Read the model definition and answer for the solid it produces. Units are mm, in the model's axes. A direction names the side the tool comes from. Give positions to 0.01 mm unless a question says otherwise; leave off trailing zeros. Loops run counter-clockwise (first coordinate to the right, second up) from the corner with the lowest first, then second, coordinate; pieces in that order, holes last. Notation, with made-up numbers: (36.5, 84.25) - (76.5, 84.25) arc R30 cw to (76.5, 122.25) - close; hole circle Ø6 at (82, 3.5). An arc over 180 degrees is marked (long way). Put each result on its own line as item: value. Start each with the question number.
1. A cutting plane is placed at C-C, the plane y = 5.5. Determine the outline of the cut face in (x, z), plus the area to 3 significant figures.
2. Consider L1, parallel to Z at x = 5, y = 1.5; L2, parallel to X at y = -0.5, z = 6; L3, parallel to X at y = -10.5, z = -11. Determine where each line is inside the solid, lowest interval first. Write a range as from..to.
3. A cutting plane is placed at D-D, the plane x = 13. Determine the outline of the cut face in (y, z), plus the area to 3 significant figures.
4. For faces 4 (the cylindrical face through (77.91, 0.21, -29.19)), 5 (the cylindrical face through (37.73, -0.07, 4.06)), 6 (the flat face through (23, -4, 0)), determine the directions among +Z, -Z, +X, -X, +Y, -Y from which every point of the face is accessible in a straight line to the end or side of a thin tool.
5. A cutting plane is placed at B-B, the plane y = 0. Determine the outline of the cut face in (x, z).
6. A cutting plane is placed at A-A, the plane x = 26.5. Determine the outline of the cut face in (y, z), plus the area to 3 significant figures.
7. Given pin 1 Ø2 at (y, z) = (-4.5, -28) entering from +X; pin 2 Ø3 at (x, y) = (59.5, -10) entering from -Z; pin 3 Ø5 at (y, z) = (-12, -5.5) entering from +X, each flat-ended and moving along its own axis, determine where each tip first touches the part or whether it passes through.
8. For a pull along X with two mould halves and no side action, classify faces 1 (the flat face through (60.66, -0.21, -17.47)), 2 (the flat face through (25, 3, 4)), 3 (the flat face through (43, -15, 2)) as released by +X, released by -X, zero draft, split by the parting line, or undercut.
```python
from build123d import *

# Parameters (mm, degrees)
F1_DEPTH    = 15
F3_DEPTH    = 43.4455230334
F5_D        = 4
F6_T1_DEPTH = 78.9897948557
F6_T3_DEPTH = 58
F7_SIZE     = 5


# Not quite as in the source:
# - a fillet or chamfer that OpenCascade refuses, or shapes differently, is made with other operations: its cross-section is extruded or revolved along the edge and cut away or added


with BuildPart() as f1:
    # F0 (on Front) → F1 (new body, symmetric)
    with BuildSketch(Plane.XZ):
        Polygon((-0.2695387348, 8), (0, 0), (46, 0), (75.7414862046, -35.4445230334), (81.8698417496, -30.3022221559), (49.7304612652, 8), align=None)
    extrude(amount=F1_DEPTH, both=True)

    # F2 (on face) → F3 (cut, through all)
    with BuildSketch(Plane.XY.offset(8)):
        with BuildLine():
            ThreePointArc((14.7304612652, 3), (11.7304612652, 0), (14.7304612652, -3))
            Line((14.7304612652, -3), (34.7304612652, -3))
            ThreePointArc((34.7304612652, -3), (37.7304612652, 0), (34.7304612652, 3))
            Line((34.7304612652, 3), (14.7304612652, 3))
        make_face()
    extrude(amount=-F3_DEPTH, mode=Mode.SUBTRACT)

    # F5 (through all)
    with Locations(Plane(origin=(33.1222636313, 0, 27.7928791968), x_dir=(0, 1, 0), z_dir=(0.7660444431, 0, 0.6427876097))):
        with Locations((0, -40.8377687803), (0, -60.8377687803)):
            Hole(F5_D / 2)

    # F6: fillet of radius 10 on 2 edges, made by hand

    # F6_s2 → F6_t1 (cut)
    with BuildSketch(Plane.XZ.offset(-39.4948974278)):
        with BuildLine():
            ThreePointArc((75.7414862046, -35.4445230334), (77.9104912295, -29.0903052725), (75.5718351227, -22.7965501322))
            Line((75.5718351227, -22.7965501322), (81.8698417496, -30.3022221559))
            Line((81.8698417496, -30.3022221559), (75.7414862046, -35.4445230334))
        make_face()
    extrude(amount=F6_T1_DEPTH, mode=Mode.SUBTRACT)

    # F6_s4 → F6_t3 (cut)
    with BuildSketch(Plane(origin=(7.8427970084, 0, 6.5808880771), x_dir=(0, 1, 0), z_dir=(0.7660444431, 0, 0.6427876097))):
        with BuildLine():
            ThreePointArc((-15, -65.8377687803), (-12.0710678119, -72.9088365922), (-5, -75.8377687803))
            Line((-5, -75.8377687803), (-15, -75.8377687803))
            Line((-15, -75.8377687803), (-15, -65.8377687803))
        make_face()
    extrude(amount=F6_T3_DEPTH, mode=Mode.SUBTRACT)

    # F7
    f7_edges = [f1.edges().sort_by_distance(p)[0] for p in [
        (-0.134769, -15, 4),
        (-0.134769, 15, 4),
    ]]
    chamfer(f7_edges, length=F7_SIZE)


solid = f1.part
```
Return value:
1. outline: (-0.27, 8) - (0, 0) - (46, 0) - (75.74, -35.44) arc R10 ccw to (75.57, -22.8) - (49.73, 8) - close
1. area: 749 mm2
2. L1: z = 0..8
2. L2: x = -0.2..11.77, 37.69..51.41
2. L3: x = 55.23..65.67
3. outline: (-15, 0) - (-2.45, 0) - (-2.45, 8) - (-15, 8) - close; (2.45, 0) - (15, 0) - (15, 8) - (2.45, 8) - close
3. area: 201 mm2
4. face 4: +X, +Y, -Y
4. face 5: +Z, -Z
4. face 6: -Z, -X, +Y, -Y
5. outline: (-0.27, 8) - (0, 0) - (11.73, 0) - (11.73, 8) - close; (37.73, 0) - (46, 0) - (51.96, -7.1) - (58.09, -1.96) - (49.73, 8) - (37.73, 8) - close; (54.53, -10.17) - (64.81, -22.42) - (70.94, -17.28) - (60.66, -5.02) - close; (67.39, -25.49) - (75.74, -35.44) arc R10 ccw to (75.57, -22.8) - (73.51, -20.34) - close
6. outline: (-15, 0) - (-3, 0) - (-3, 8) - (-15, 8) - close; (3, 0) - (15, 0) - (15, 8) - (3, 8) - close
6. area: 192 mm2
7. pin 1: stops at x = 77.91
7. pin 2: stops at z = -17.88
7. pin 3: stops at x = 63.16
8. face 1: released by -X
8. face 2: undercut
8. face 3: zero draft
